For this review, take the finished solid that the model builds, in its own axes (mm). Face numbers are marked on the shaded views. A direction names the side the tool comes from. Coordinates: 2 decimals unless noted, no trailing zeros. Write each loop counter-clockwise with the first axis right and the second up, starting at its lowest first coordinate (ties: lowest second). Pieces come first, ordered by that corner, then holes. Notation, with made-up numbers: (13, -18) -> (48, -18) arc R29 ccw to (48, 14) -> close; hole circle Ø6 at (39, -38.75). An arc over 180 degrees is marked (long way). Put each result on its own line as item: value. Start each with the question number.
Item 1: Consider section B-B on x = -5. Give the boundary of the cut face in (y, z).
Item 2: Consider section A-A on y = -2.75. Give the boundary of the cut face in (x, z), and give its area (3 significant figures).
Item 3: Consider section D-D on z = 7. Give the number of separate pieces and of enclosed holes in the cut face, and give its area (3 significant figures).
Item 4: To check wall thickness, follow L1, parallel to X at y = -11, z = 0; L2, parallel to X at y = -11, z = -12.25; L3, parallel to Y at x = -28, z = 3. State the ranges of each line that lie inside material, in increasing order.
Item 5: Insertion check: P1, Ø3.5, axis at y = -13, z = 4, coming from the +X side; P2, Ø1.5, axis at x = 13.5, z = -1, coming from the -Y side; P3, Ø2.5, axis at x = -4.5, y = -5.5, coming from the +Z side. Each pin has a flat end and moves straight along its axis. Give the tip position at first contact, or say it passes through.
Item 6: For the marked faces 1, 2 and 3, list the 3-axis set-ups (+Z, -Z, +X, -X, +Y, -Y) from which the entire face can be reached by the end or side of a thin tool; tool diameter is ignored.
Item 7: The part is to be moulded in two halves that separate along X. For the marked faces 4, 5, 6 and 7, say which applies: +X half, -X half, draft (parallel to the pull), parting line (faces both ways), or undercut.
Item 8: Consider section C-C on z = -10.25. Give the boundary of the cut face in (x, y).
```python
from build123d import *

# Parameters (mm, degrees)
BOSS_EXTRUDE1_DEPTH      = 10
BOSS_EXTRUDE1_DEPTH_BACK = 15
SKETCH2_R                = 1.2
CUT_EXTRUDE1_DEPTH       = 39.794329483
LPATTERN1_COUNT          = 9
LPATTERN1_PITCH          = 8
CUT_EXTRUDE2_START       = -10
SKETCH3_W                = 6
SKETCH3_H                = 3
CUT_EXTRUDE2_DEPTH       = 10
LPATTERN2_COUNT          = 8
LPATTERN2_PITCH          = 8
LPATTERN2_COUNT_DIR2     = 2
LPATTERN2_PITCH_DIR2     = 8


with BuildPart() as part:
    # Sketch1 → Boss-Extrude1 (new, two sides: drawn at the far end of the back side and taken through both)
    with BuildSketch(Plane.XY.offset(-BOSS_EXTRUDE1_DEPTH_BACK)):
        Polygon((-32, 0), (32, 0), (32, -8), (24, -8), (24, -16), (16, -16), (16, -8), (8, -8), (8, -16), (0, -16), (0, -8), (-8, -8), (-8, -16), (-16, -16), (-16, -8), (-24, -8), (-24, -16), (-32, -16), align=None)
    extrude(amount=BOSS_EXTRUDE1_DEPTH + BOSS_EXTRUDE1_DEPTH_BACK)

    # Sketch2 → Cut-Extrude1 (cut, through all)
    with BuildSketch(Plane(origin=(0, 0, 0), x_dir=(1, 0, 0), z_dir=(0, 1, 0))):
        with Locations((-32, 0)):
            Circle(SKETCH2_R)
    cut_extrude1 = extrude(amount=-CUT_EXTRUDE1_DEPTH, mode=Mode.SUBTRACT)

    # LPattern1: Cut-Extrude1 ×9
    with Locations(*[(i * LPATTERN1_PITCH, 0, 0) for i in range(1, LPATTERN1_COUNT)]):
        add(cut_extrude1, mode=Mode.SUBTRACT)

    # Sketch3 → Cut-Extrude2 (cut)
    with BuildSketch(Plane.XY.offset(10).offset(CUT_EXTRUDE2_START)):
        with Locations((-28, -5.5)):
            Rectangle(SKETCH3_W, SKETCH3_H)
    cut_extrude2 = extrude(amount=CUT_EXTRUDE2_DEPTH, mode=Mode.SUBTRACT)

    # LPattern2: Cut-Extrude2 8 × 2
    with Locations(*[(i * LPATTERN2_PITCH, -j * LPATTERN2_PITCH_DIR2, 0) for i in range(LPATTERN2_COUNT) for j in range(LPATTERN2_COUNT_DIR2) if (i, j) != (0, 0)]):
        add(cut_extrude2, mode=Mode.SUBTRACT)


solid = part.part
```
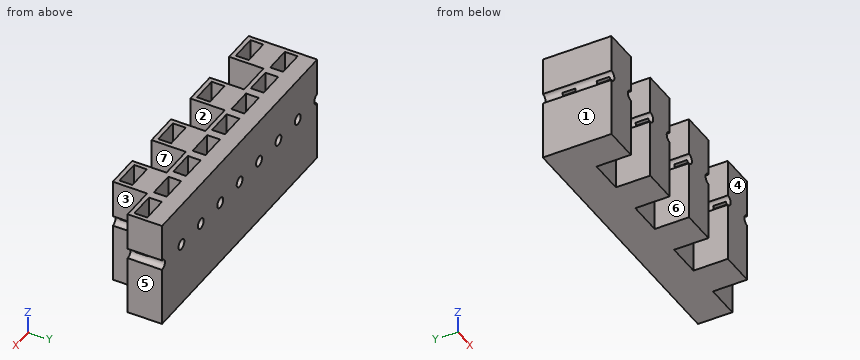
Return value:
1. outline: (-8, -15) -> (0, -15) -> (0, 10) -> (-4, 10) -> (-4, 0) -> (-7, 0) -> (-7, 10) -> (-8, 10) -> close
2. outline: (-32, -15) -> (32, -15) -> (32, -1.2) arc R1.2 cw to (32, 1.2) -> (32, 10) -> (-32, 10) -> (-32, 1.2) arc R1.2 cw to (-32, -1.2) -> close; hole circle Ø2.4 at (-24, 0); hole circle Ø2.4 at (-16, 0); hole circle Ø2.4 at (-8, 0); hole circle Ø2.4 at (0, 0); hole circle Ø2.4 at (8, 0); hole circle Ø2.4 at (16, 0); hole circle Ø2.4 at (24, 0)
2. area: 1,560 mm^2
3. separate pieces: 1
3. enclosed holes: 12
3. area: 552 mm^2
4. L1: -30.8 to -25.2, -14.8 to -9.2, 1.2 to 6.8, 17.2 to 22.8
4. L2: -32 to -24, -16 to -8, 0 to 8, 16 to 24
4. L3: -16 to -15, -12 to -7, -4 to 0
5. P1: x = 24
5. P2: y = -8
5. P3: z = 0
6. face 1: +Z, -Z, -X, +Y, -Y
6. face 2: +Z, -Z, -Y
6. face 3: +Z, -Z, +X, -Y
7. face 4: draft
7. face 5: +X half
7. face 6: undercut
7. face 7: undercut
8. outline: (-32, -16) -> (-24, -16) -> (-24, -8) -> (-16, -8) -> (-16, -16) -> (-8, -16) -> (-8, -8) -> (0, -8) -> (0, -16) -> (8, -16) -> (8, -8) -> (16, -8) -> (16, -16) -> (24, -16) -> (24, -8) -> (32, -8) -> (32, 0) -> (-32, 0) -> close
